Part model, mm, in its own coordinate system. Face numbers are marked on the shaded views. A direction names the side the tool comes from. Coordinates: 2 decimals unless noted, no trailing zeros. Order: outer loops, then holes, each group sorted by start corner. A loop starts at its lowest first (then second) coordinate and runs counter-clockwise, first axis right, second up.
from build123d import *

# Parameters (mm, degrees)
SKETCH1_R                   = 35
BOSS_EXTRUDE1_DEPTH         = 10
SKETCH2_R                   = 23
BOSS_EXTRUDE2_DEPTH         = 7
BOSS_EXTRUDE3_DEPTH         = 4
SKETCH4_R                   = 1.5
CUT_EXTRUDE1_DEPTH          = 4
FILLET1_R                   = 2
FILLET1_OF_MIRROR1_R        = 2
SKETCH5_W                   = 2
SKETCH5_H                   = 6
BOSS_EXTRUDE4_DEPTH         = 10
FILLET2_RADIUS              = 1
FILLET2_LENGTH              = 10
FILLET2_OF_MIRROR2_2_RADIUS = 1
FILLET2_OF_MIRROR2_2_LENGTH = 10
SKETCH6_R                   = 15
CUT_EXTRUDE2_DEPTH          = 10


with BuildPart() as part:
    # Sketch1 → Boss-Extrude1 (new body)
    with BuildSketch(Plane.XY):
        Circle(SKETCH1_R)
    extrude(amount=BOSS_EXTRUDE1_DEPTH)

    # Sketch2 → Boss-Extrude2 (add)
    with BuildSketch(Plane.XY.offset(10)):
        Circle(SKETCH2_R)
    extrude(amount=BOSS_EXTRUDE2_DEPTH)

    # Sketch3 → Boss-Extrude3 (add)
    with BuildSketch(Plane(origin=(0, 13, 0), x_dir=(1, 0, 0), z_dir=(0, 1, 0))):
        Polygon((35, -17), (-35, -17), (-41.135319403, -22.148144248), (-41.135319403, -27.148144248), (-23, -42.36548407), (23, -42.36548407), (41.135319403, -27.148144248), (41.135319403, -22.148144248), align=None)
    boss_extrude3 = extrude(amount=-BOSS_EXTRUDE3_DEPTH)

    # Sketch4 → Cut-Extrude1 (cut)
    with BuildSketch(Plane(origin=(0, 13, 0), x_dir=(1, 0, 0), z_dir=(0, 1, 0))):
        with Locations(Location((-38.135319403, -24.648144248, 0), (0, 0, 270))):
            Circle(SKETCH4_R)
        with Locations(Location((38.135319403, -24.648144248, 0), (0, 0, 90))):
            Circle(SKETCH4_R)
    cut_extrude1 = extrude(amount=-CUT_EXTRUDE1_DEPTH, mode=Mode.SUBTRACT)

    # Fillet1
    fillet1_edges = [part.edges().sort_by_distance(p)[0] for p in [
        (23, 11, 42.36548407),
        (-23, 11, 42.36548407),
        (-41.135319403, 11, 27.148144248),
        (-41.135319403, 11, 22.148144248),
        (41.135319403, 11, 22.148144248),
        (41.135319403, 11, 27.148144248),
    ]]
    fillet(fillet1_edges, radius=FILLET1_R)

    # Mirror1: Boss-Extrude3, Cut-Extrude1 across plane
    add(boss_extrude3.mirror(Plane.ZX))
    add(cut_extrude1.mirror(Plane.ZX), mode=Mode.SUBTRACT)

    # Fillet1 of Mirror1
    fillet1_of_mirror1_edges = [part.edges().sort_by_distance(p)[0] for p in [
        (23, -11, 42.36548407),
        (-23, -11, 42.36548407),
        (-41.135319403, -11, 27.148144248),
        (-41.135319403, -11, 22.148144248),
        (41.135319403, -11, 22.148144248),
        (41.135319403, -11, 27.148144248),
    ]]
    fillet(fillet1_of_mirror1_edges, radius=FILLET1_OF_MIRROR1_R)

    # Sketch5 → Boss-Extrude4 (add)
    with BuildSketch(Plane.XY.offset(17)):
        with Locations((0, 16)):
            Rectangle(SKETCH5_W, SKETCH5_H)
    boss_extrude4 = extrude(amount=BOSS_EXTRUDE4_DEPTH)

    # Fillet2: full round fillet: the end face becomes a half cylinder, R = half its width
    fillet2_face = Plane((0, 19, 22), x_dir=(0, 0, -1), z_dir=(0, 1, 0))  # on the end face: x along it, z out of the body
    fillet2_slab = fillet2_face.offset(-FILLET2_RADIUS / 2) * Box(FILLET2_LENGTH, 2 * FILLET2_RADIUS, FILLET2_RADIUS, mode=Mode.PRIVATE)  # the body's end, R deep
    fillet2_round = Plane((0, 18, 22), x_dir=(0, 1, 0), z_dir=(0, 0, -1)) * Cylinder(FILLET2_RADIUS, FILLET2_LENGTH, mode=Mode.PRIVATE)  # its axis R under the face
    add(fillet2_slab - fillet2_round, mode=Mode.SUBTRACT)

    # Mirror2: Boss-Extrude4 across plane
    add(boss_extrude4.mirror(Plane.ZX))

    # Fillet2 of Mirror2 2: full round fillet: the end face becomes a half cylinder, R = half its width
    fillet2_of_mirror2_2_face = Plane((0, -19, 22), x_dir=(0, 0, -1), z_dir=(0, -1, 0))  # on the end face: x along it, z out of the body
    fillet2_of_mirror2_2_slab = fillet2_of_mirror2_2_face.offset(-FILLET2_OF_MIRROR2_2_RADIUS / 2) * Box(FILLET2_OF_MIRROR2_2_LENGTH, 2 * FILLET2_OF_MIRROR2_2_RADIUS, FILLET2_OF_MIRROR2_2_RADIUS, mode=Mode.PRIVATE)  # the body's end, R deep
    fillet2_of_mirror2_2_round = Plane((0, -18, 22), x_dir=(0, -1, 0), z_dir=(0, 0, -1)) * Cylinder(FILLET2_OF_MIRROR2_2_RADIUS, FILLET2_OF_MIRROR2_2_LENGTH, mode=Mode.PRIVATE)  # its axis R under the face
    add(fillet2_of_mirror2_2_slab - fillet2_of_mirror2_2_round, mode=Mode.SUBTRACT)

    # Sketch6 → Cut-Extrude2 (cut)
    with BuildSketch(Plane(origin=(0, 0, 0), x_dir=(-1, 0, 0), z_dir=(0, 0, -1))):
        Circle(SKETCH6_R)
    extrude(amount=-CUT_EXTRUDE2_DEPTH, mode=Mode.SUBTRACT)


solid = part.part
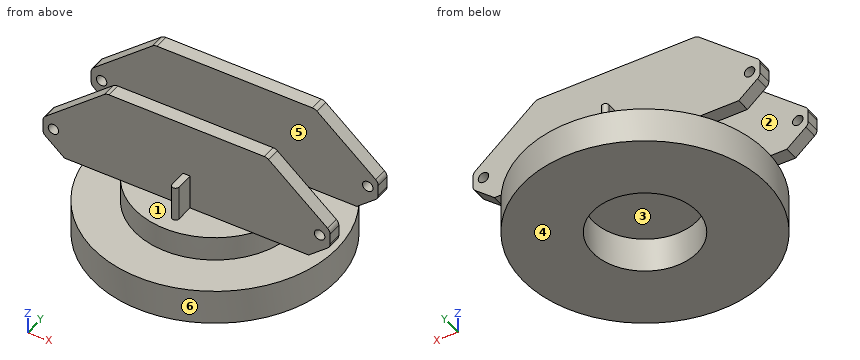
Q1. Cut at A-A on x = 24.5. Write the cut outline in (y, z) (3 decimals).
Results list:
outline: (-24.995, 0) - (24.995, 0) - (24.995, 10) - (-24.995, 10) - close; (-13, 17) - (-9, 17) - (-9, 41.107) - (-13, 41.107) - close; (9, 17) - (13, 17) - (13, 41.107) - (9, 41.107) - close
Q2. Cut at D-D on y = 0. Write the cut outline in (x, z), and give its area (3 significant figures).
Results list:
outline: (-35, 0) - (-15, 0) - (-15, 10) - (15, 10) - (15, 0) - (35, 0) - (35, 10) - (23, 10) - (23, 17) - (-23, 17) - (-23, 10) - (-35, 10) - close
area: 722 mm2
Q3. Which spindle directions (+Z, -Z, +X, -X, +Y, -Y) get a long thin tool onto all of the face, cutting with end or side? Do the marked faces 1, 2 and 3. Say none if no direction does.
Results list:
face 1: +Z, -Y
face 2: +Z, +X, -X
face 3: -Z
Q4. Pin check, flat tips, straight feed: pin 1 Ø1.5 at (y, z) = (16.5, 20) entering from -X; pin 2 Ø4 at (y, z) = (-16.5, 24) entering from +X; pin 3 Ø2 at (y, z) = (-3, 18.5) entering from -X; pin 4 Ø3 at (x, y) = (-0.5, 16) entering from +Z. Stop position of each tip, or through.
Results list:
pin 1: stops at x = -1
pin 2: stops at x = 1
pin 3: passes through
pin 4: stops at z = 27
Q5. Mould opens along Y. For the marked faces 4, 5 and 6 say: pulls with the +Y half, pulls with the -Y half, needs draft (parallel to the pull), parting line crosses it, or undercut.
Results list:
face 4: needs draft
face 5: undercut
face 6: parting line crosses it
Q6. Cut at B-B on y = 12. Write the cut outline in (x, z).
Results list:
outline: (-41.14, 23.08) arc R2 ccw to (-40.42, 21.55) - (-35, 17) - (-19.62, 17) - (-19.62, 10) - (-32.88, 10) - (-32.88, 0) - (-9, 0) - (-9, 10) - (9, 10) - (9, 0) - (32.88, 0) - (32.88, 10) - (19.62, 10) - (19.62, 17) - (35, 17) - (40.42, 21.55) arc R2 ccw to (41.14, 23.08) - (41.14, 26.22) arc R2 ccw to (40.42, 27.75) - (23.56, 41.9) arc R2 ccw to (22.27, 42.37) - (-22.27, 42.37) arc R2 ccw to (-23.56, 41.9) - (-40.42, 27.75) arc R2 ccw to (-41.14, 26.22) - close; hole circle Ø3 at (-38.14, 24.65); hole circle Ø3 at (38.14, 24.65)
Q7. Cut at C-C on x = 0. Write the cut outline in (y, z), and give its area (3 significant figures).
Results list:
outline: (-35, 0) - (-15, 0) - (-15, 10) - (15, 10) - (15, 0) - (35, 0) - (35, 10) - (23, 10) - (23, 17) - (19, 17) - (19, 27) - (13, 27) - (13, 42.37) - (9, 42.37) - (9, 17) - (-9, 17) - (-9, 42.37) - (-13, 42.37) - (-13, 27) - (-19, 27) - (-19, 17) - (-23, 17) - (-23, 10) - (-35, 10) - close
area: 1,040 mm2
Q8. Wall check: line 1 along Y through (x, z) = (5.5, 26); line 2 along Y through (x, z) = (0, 6.25); line 3 along Z through (x, y) = (-3.5, -20.5). Give the ranges that are in metal, low to high.
Results list:
line 1: y = -13 to -9, 9 to 13
line 2: y = -35 to -15, 15 to 35
line 3: z = 0 to 17
